For this review, take the finished solid that the model builds, in its own axes (mm). Give positions to 0.01 mm unless a question says otherwise; leave off trailing zeros. Order: outer loops, then holes, each group sorted by start corner. A loop starts at its lowest first (then second) coordinate and runs counter-clockwise, first axis right, second up. Notation, with made-up numbers: (60, 81.25) - (86, 81.25) arc R26 cw to (86, 115.25) - close; hole circle Ø5 at (-24.75, -10). An arc over 180 degrees is marked (long way). Use a Markdown table: item, result. Add a question column.
1) Clearance check with a flat-ended pin moving along its axis: P1, Ø1.5, axis at y = 21, z = -2, coming from the -X side. State where the tip first meets the part, or that it passes through.
2) Wall thickness on L1, parallel to Y at x = -12.5, z = -1.1; L2, parallel to X at y = 20.5, z = -0.55: over which ranges is each line inside the solid? List them lowest first.
3) We need section B-B on y = 20.5. Write out the cut boundary in (x, z), then the cut area to 3 significant figures.
4) We need section A-A on x = -9.5. Write out the cut boundary in (y, z), then the cut area to 3 significant figures.
5) We need section C-C on z = -2.2. Write out the cut boundary in (x, y), then the cut area to 3 significant figures.
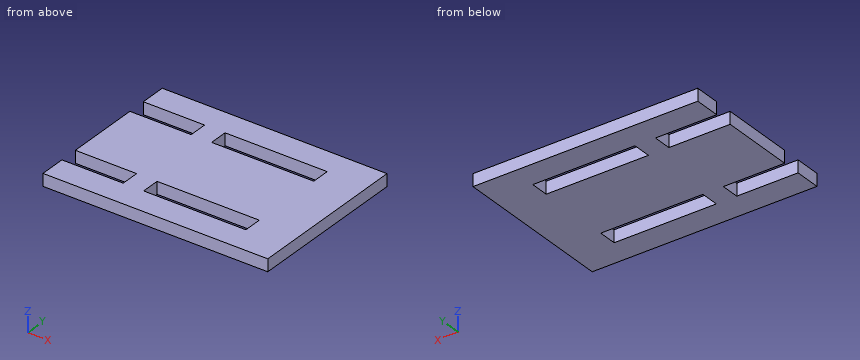
```python
from build123d import *

# Parameters (mm, degrees)
SKETCH1_W           = 25
SKETCH1_H           = 4.5
BOSS_EXTRUDE1_DEPTH = 3


with BuildPart() as part:
    # Sketch1 → Boss-Extrude1 (new body)
    with BuildSketch(Plane.XY):
        Polygon((-33.65, -10.85), (21.35, -10.85), (21.35, 29.15), (-33.65, 29.15), (-33.65, 22.8), (-18.65, 22.8), (-18.65, 18.3), (-33.65, 18.3), (-33.65, 0), (-18.65, 0), (-18.65, -4.5), (-33.65, -4.5), align=None)
        with Locations((-1.15, -2.25)):
            Rectangle(SKETCH1_W, SKETCH1_H, mode=Mode.SUBTRACT)
        with Locations((-1.15, 20.55)):
            Rectangle(SKETCH1_W, SKETCH1_H, mode=Mode.SUBTRACT)
    extrude(amount=-BOSS_EXTRUDE1_DEPTH)


solid = part.part
```
Checked values:
| question | item | result |
|---|---|---|
| 1 | P1 | x = -18.65 |
| 2 | L1 | -10.85 to -4.5, 0 to 18.3, 22.8 to 29.15 |
| 2 | L2 | -18.65 to -13.65, 11.35 to 21.35 |
| 3 | outline | (-18.65, -3) - (-13.65, -3) - (-13.65, 0) - (-18.65, 0) - close; (11.35, -3) - (21.35, -3) - (21.35, 0) - (11.35, 0) - close |
| 3 | area | 45.0 mm² |
| 4 | outline | (-10.85, -3) - (-4.5, -3) - (-4.5, 0) - (-10.85, 0) - close; (0, -3) - (18.3, -3) - (18.3, 0) - (0, 0) - close; (22.8, -3) - (29.15, -3) - (29.15, 0) - (22.8, 0) - close |
| 4 | area | 93.0 mm² |
| 5 | outline | (-33.65, -10.85) - (21.35, -10.85) - (21.35, 29.15) - (-33.65, 29.15) - (-33.65, 22.8) - (-18.65, 22.8) - (-18.65, 18.3) - (-33.65, 18.3) - (-33.65, 0) - (-18.65, 0) - (-18.65, -4.5) - (-33.65, -4.5) - close; hole (-13.65, -4.5) - (11.35, -4.5) - (11.35, 0) - (-13.65, 0) - close; hole (-13.65, 18.3) - (11.35, 18.3) - (11.35, 22.8) - (-13.65, 22.8) - close |
| 5 | area | 1,840 mm² |
